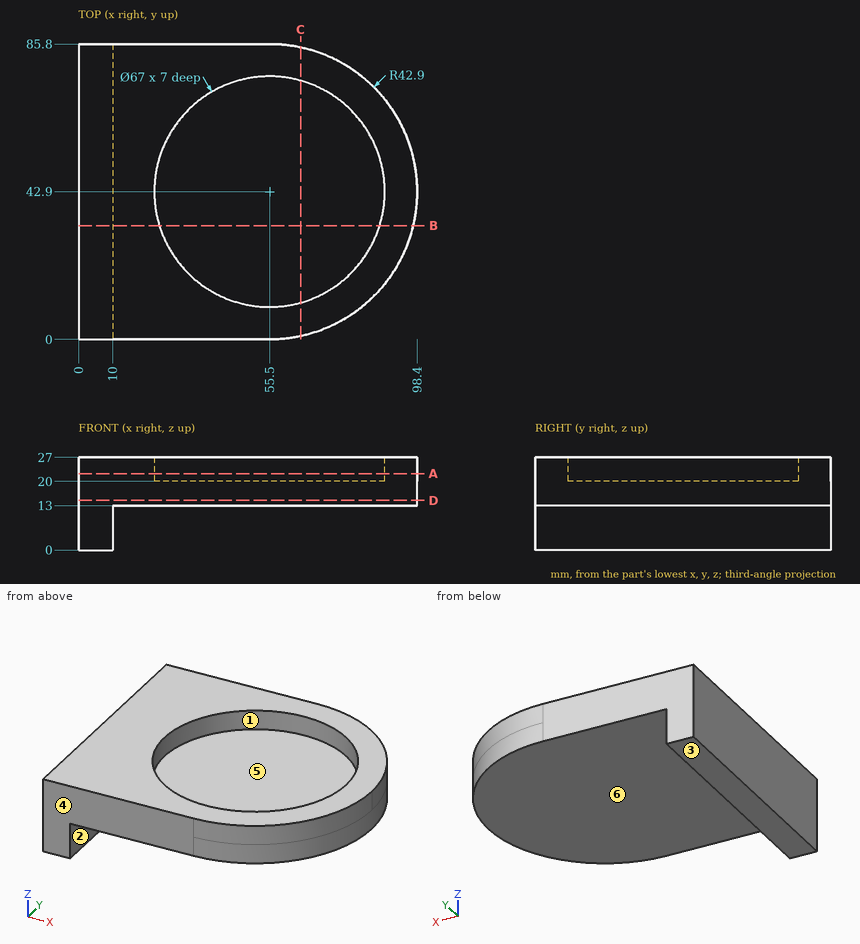
Design review of the part shown in the three views and the two pictorial views. Dimensions are in mm from the part's minimum x, y and z. A direction names the side the tool comes from. Give positions to 0.01 mm unless a question says otherwise; leave off trailing zeros. Write each loop counter-clockwise with the first axis right and the second up, starting at its lowest first coordinate (ties: lowest second). Pieces come first, ordered by that corner, then holes.
Item 1: Machinability: for the marked faces 4, 5 and 6, which of the approach directions +Z, -Z, +X, -X, +Y, -Y give a long, thin tool a straight path to every point of the face, cutting with its end or side? Answer none if there is none.
Item 2: Take a section at B-B (y = 33). Give the boundary of the cut face in (x, z), and give its area (3 significant figures).
Item 3: Wall thickness on probe 1 along Y at (x, z) = (55.5, 25); probe 2 along X at (y, z) = (24, 2.25); probe 3 along Z at (x, y) = (56, 19): over which ranges is each line inside the solid? List them lowest first.
Item 4: The part is to be moulded in two halves that separate along X. For the marked faces 1, 2 and 3, say which applies: +X half, -X half, draft (parallel to the pull), parting line (faces both ways), or undercut.
Item 5: Take a section at A-A (z = 22.25). Give the boundary of the cut face in (x, y), and give its area (3 significant figures).
Item 6: Insertion check: P1, Ø10, axis at y = 43.5, z = 9.5, coming from the +X side. The pin has a flat end and moves straight along its axis. Give the tip position at first contact, or say it passes through.
Item 7: Take a section at C-C (x = 64.5). Give the boundary of the cut face in (y, z), and give its area (3 significant figures).
Item 8: Take a section at D-D (z = 14.5). Give the boundary of the cut face in (x, y), and give its area (3 significant figures).
Established:
1. face 4: +Z, -Z, +X, -X, -Y
1. face 5: +Z
1. face 6: -Z, +X, +Y, -Y
2. outline: (0, 0) - (10, 0) - (10, 13) - (97.24, 13) - (97.24, 27) - (87.5, 27) - (87.5, 20) - (23.5, 20) - (23.5, 27) - (0, 27) - close
2. area: 1,040 mm2
3. probe 1: y = 0 to 9.4, 76.4 to 85.8
3. probe 2: x = 0 to 10
3. probe 3: z = 13 to 20
4. face 1: undercut
4. face 2: +X half
4. face 3: draft
5. outline: (0, 0) - (55.5, 0) arc R42.9 ccw to (55.5, 85.8) - (0, 85.8) - close; hole circle Ø67 at (55.5, 42.9)
5. area: 4,130 mm2
6. P1: stops at x = 98.4
7. outline: (0.95, 13) - (84.85, 13) - (84.85, 27) - (75.17, 27) - (75.17, 20) - (10.63, 20) - (10.63, 27) - (0.95, 27) - close
7. area: 723 mm2
8. outline: (0, 0) - (55.5, 0) arc R42.9 ccw to (55.5, 85.8) - (0, 85.8) - close
8. area: 7,650 mm2
